Design review of the part built by this model. Coordinates are the model's own, in mm. Face numbers are marked on the shaded views. A direction names the side the tool comes from. Round coordinates to 2 decimals unless told otherwise and drop trailing zeros. Order: outer loops, then holes, each group sorted by start corner. A loop starts at its lowest first (then second) coordinate and runs counter-clockwise, first axis right, second up. Notation, with made-up numbers: M 20.25,70.5 L 72.25,70.5 A17 ccw 72.25,101.5 Z; hole C 51.5,-2 d9. An arc over 180 degrees is marked long. Write each question's results on one line, items separated by ' | '. Start each with the question number.
Item 1: Take a section at D-D, the plane z = -15. Write out the cut boundary in (x, y), plus the area to 3 significant figures.
Item 2: Take a section at B-B, the plane x = 14.5. Write out the cut boundary in (y, z).
Item 3: Take a section at A-A, the plane z = 0. Write out the cut boundary in (x, y), plus the area to 3 significant figures.
Item 4: Machinability: for the marked faces 1, 2 and 3, which of the approach directions +Z, -Z, +X, -X, +Y, -Y give a long, thin tool a straight path to every point of the face, cutting with its end or side? Answer none if there is none.
Item 5: Wall thickness on line 1 (Y direction, x = 10.25, z = 0); line 2 (X direction, y = -7.25, z = -12); line 3 (Z direction, x = 1, y = -3.25): over which ranges is each line inside the solid? List them lowest first. Write a range as [from, to].
Item 6: The part is to be moulded in two halves that separate along Y. For the marked faces 4, 5, 6 and 7, say which applies: +Y half, -Y half, draft (parallel to the pull), parting line (faces both ways), or undercut.
Item 7: Clearance check with flat-ended pins moving along their axes: pin 1 (5.5 mm diameter, centred on y = 0, z = -15, fed in from +X); pin 2 (8.5 mm diameter, centred on y = 0, z = 0, fed in from +X); pin 3 (8 mm diameter, centred on y = 0, z = 0, fed in from -X); pin 4 (4 mm diameter, centred on x = 7, y = 0, fed in from +Z). State where each tip first meets the part, or that it passes through.
Item 8: Take a section at C-C, the plane y = 0. Count the separate pieces of the cut face and the enclosed holes in it, plus the area to 3 significant figures.
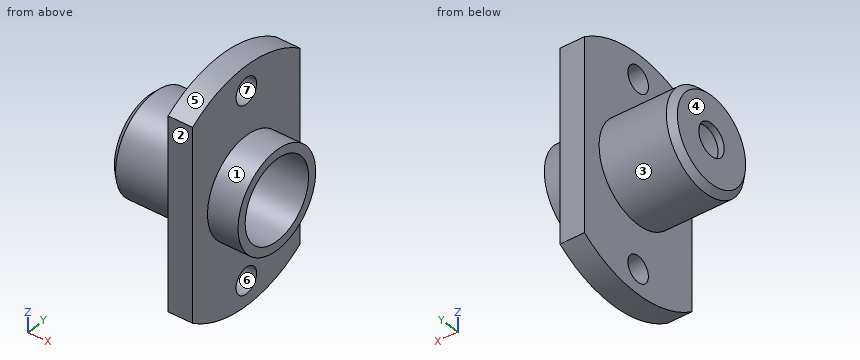
```python
from build123d import *

# Parameters (mm, degrees)
F2_R     = 2.1
F3_DEPTH = 9.001
F4_SIZE  = 1


# Not quite as in the source:
# - a feature names something its author has since deleted; it is built from what else it names


with BuildPart() as f1:
    # F0 (on Front) → F1 (revolve)
    with BuildSketch(Plane.XZ):
        Polygon((0, 6.5), (20, 6.5), (20, 7.95), (15, 7.95), (15, 19), (11, 19), (11, 8), (-1, 8), (-1, 2.6), (0, 2.6), align=None)
    revolve(axis=Axis((12.5816260299, 0, 0), (1, 0, 0)))

    # F2 (on face) → F3 (cut, through all)
    with BuildSketch(Plane(origin=(11, 0, 0), x_dir=(0, -1, 0), z_dir=(-1, 0, 0))):
        with Locations((0, 15)):
            Circle(F2_R)
        with Locations((0, -15)):
            Circle(F2_R)
        with BuildLine():
            Line((-11, -15.4919333848), (-11, 15.4919333848))
            ThreePointArc((-11, 15.4919333848), (-19, 0), (-11, -15.4919333848))
        make_face()
        with BuildLine():
            ThreePointArc((19, 0), (16.8819430161, 8.7177978871), (11, 15.4919333848))
            Line((11, 15.4919333848), (11, -15.4919333848))
            ThreePointArc((11, -15.4919333848), (16.8819430161, -8.7177978871), (19, 0))
        make_face()
    extrude(amount=-F3_DEPTH, mode=Mode.SUBTRACT)

    # F4
    f4_edges = [f1.edges().sort_by_distance(p)[0] for p in [
        (-1, 0, -8),
    ]]
    chamfer(f4_edges, length=F4_SIZE)


solid = f1.part
```
Results list:
1) outline: M 11,-11 L 15,-11 L 15,-2.1 L 11,-2.1 Z; M 11,2.1 L 15,2.1 L 15,11 L 11,11 Z | area: 71.2 mm²
2) outline: M -11,-15.49 A19 ccw 11,-15.49 L 11,15.49 A19 ccw -11,15.49 Z; hole C 0,0 d13; hole C 0,-15 d4.2; hole C 0,15 d4.2
3) outline: M -1,-7 L 0,-8 L 11,-8 L 11,-11 L 15,-11 L 15,-7.95 L 20,-7.95 L 20,-6.5 L 0,-6.5 L 0,-2.6 L -1,-2.6 Z; M -1,2.6 L 0,2.6 L 0,6.5 L 20,6.5 L 20,7.95 L 15,7.95 L 15,11 L 11,11 L 11,8 L 0,8 L -1,7 Z | area: 93.3 mm²
4) face 1: +X | face 2: +Z, -Z, +X, -X, -Y | face 3: -X
5) line 1: [-8, -6.5], [6.5, 8] | line 2: [11, 15] | line 3: [-7.31, -5.63], [5.63, 7.31]
6) face 4: draft | face 5: parting line | face 6: undercut | face 7: undercut
7) pin 1: x = 15 | pin 2: x = 0 | pin 3: x = -1 | pin 4: z = 8
8) separate pieces: 4 | enclosed holes: 0 | area: 124 mm²
